Drawing for the job (mm, zero at the part's lowest x, y, z). Give positions to 0.01 mm unless a question says otherwise; leave off trailing zeros. Loops run counter-clockwise (first coordinate to the right, second up) from the corner with the lowest first, then second, coordinate; pieces in that order, holes last.
1) Wall check: line 1 (Y direction, x = 103, z = 2.75); line 2 (Z direction, x = 15.5, y = 8); line 3 (X direction, y = 25.5, z = 9.5). Give the ranges that are in metal, low to high.
2) Band-saw the part on C-C on z = 5.5. List the corners of the cut face in (x, y).
3) Flat gauge pins, fed straight in: P1, Ø4, axis at x = 93, z = 4.5, coming from the +Y side; P2, Ø2, axis at x = 41, z = 8.5, coming from the -Y side; P3, Ø5, axis at y = 13, z = 3, coming from the -X side. Where does each tip first touch, or does it go through?
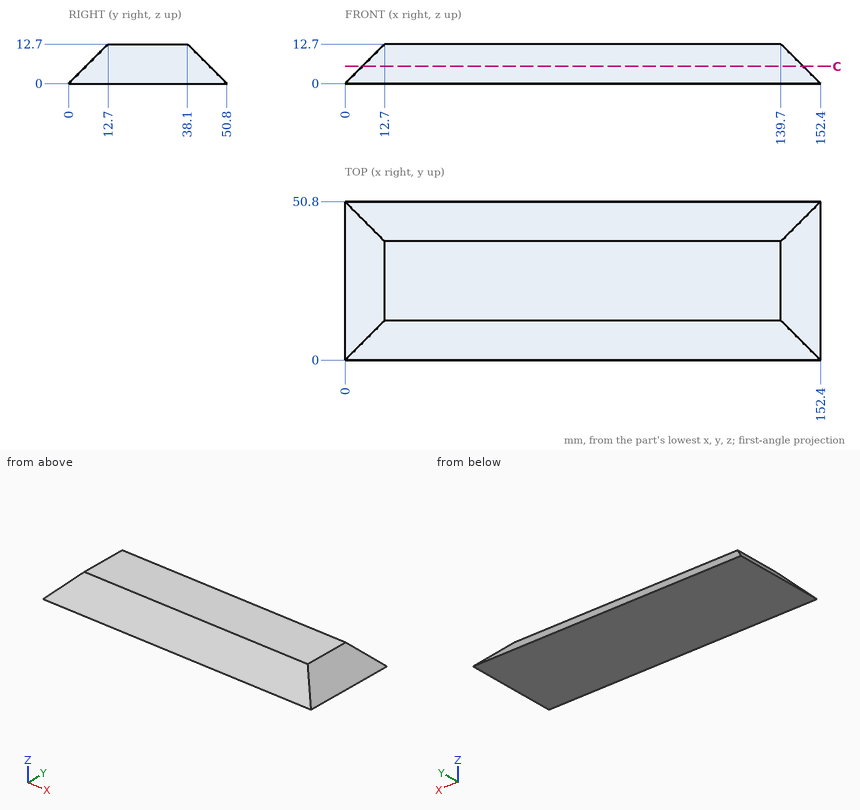
Findings below:
1. line 1: y = 2.75 to 48.05
1. line 2: z = 0 to 8
1. line 3: x = 9.5 to 142.9
2. outline: (5.5, 5.5) - (146.9, 5.5) - (146.9, 45.3) - (5.5, 45.3) - close
3. P1: stops at y = 48.3
3. P2: stops at y = 7.5
3. P3: stops at x = 0.5
